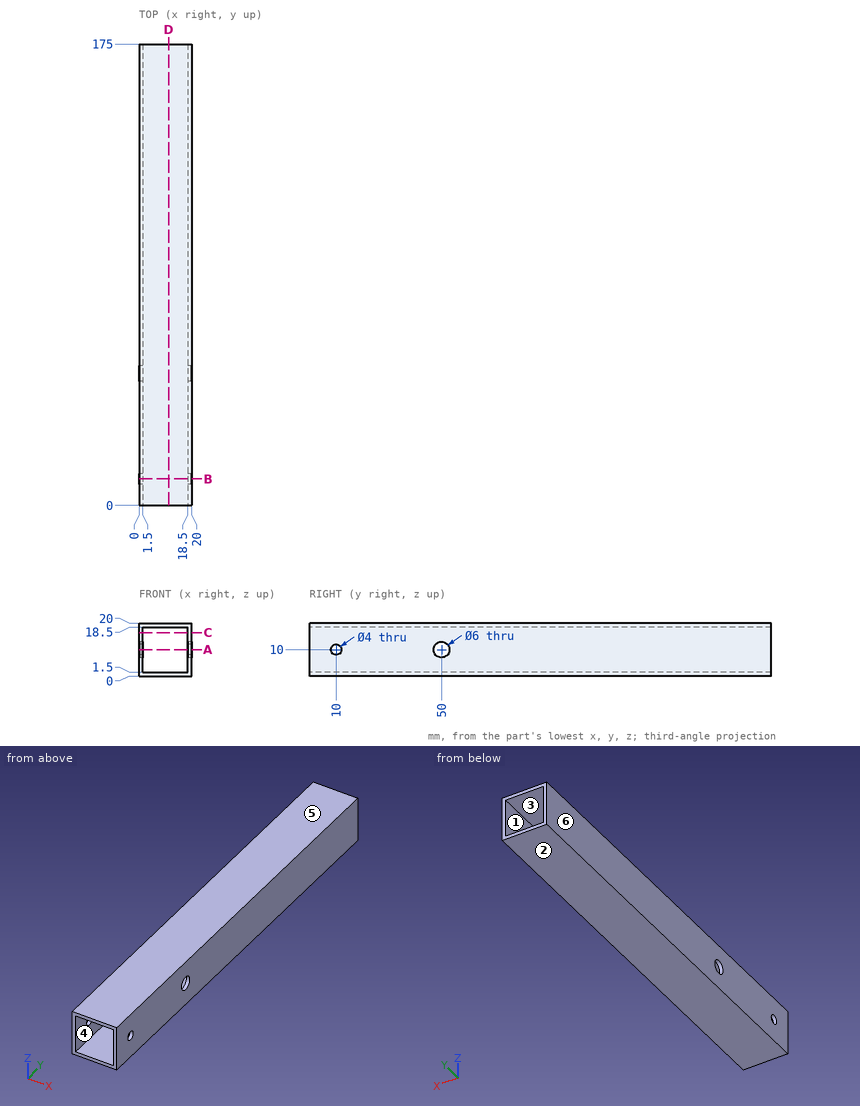
Can you work these out from the drawing? Everything is in mm from the part's minimum corner. A direction names the side the tool comes from. Coordinates: 2 decimals unless noted, no trailing zeros. Loops run counter-clockwise (first coordinate to the right, second up) from the corner with the lowest first, then second, coordinate; pieces in that order, holes last. Notation, with made-up numbers: M 2.25,-24 L 33.25,-24 A10 ccw 33.25,-19 Z; hole C 73.25,87 d10. An arc over 180 degrees is marked long. Put each result on its own line as item: value. Start each with the question number.
(1) Thinking about a two-plate mould opening in Z: for the marked faces 3, 4, 5 and 6, which applies, pulls with the +Z half, pulls with the -Z half, needs draft (parallel to the pull), parting line crosses it, or undercut?
(2) I need wall thicknesses on line 1 (Z direction, x = 0.3, y = 50); line 2 (Z direction, x = 1.75, y = 120). Which ranges of each line are inside material? Lowest first, please. Write a range as from..to.
(3) Suppose I cut it at A-A on z = 10. Please give me the cut outline in (x, y), then the cut area to 3 significant figures.
(4) Suppose I cut it at B-B on y = 10. Please give me the cut outline in (x, z), then the cut area to 3 significant figures.
(5) Suppose I cut it at C-C on z = 16.5. Please give me the cut outline in (x, y).
(6) Suppose I cut it at D-D on x = 11.25. Please give me the cut outline in (y, z), then the cut area to 3 significant figures.
(7) For the marked faces 1 and 2, which set-ups out of +Z, -Z, +X, -X, +Y, -Y let a thin tool reach every point of the face, with its end or its side?
(8) Will this pin go through, and if not, where does the flat tip stop? P1, Ø3.5, axis at y = 10, z = 10, coming from the +X side.
Solutions:
1. face 3: undercut
1. face 4: undercut
1. face 5: pulls with the +Z half
1. face 6: needs draft
2. line 1: z = 0..7, 13..20
2. line 2: z = 0..1.5, 18.5..20
3. outline: M 0,0 L 1.5,0 L 1.5,8 L 0,8 Z; M 0,12 L 1.5,12 L 1.5,47 L 0,47 Z; M 0,53 L 1.5,53 L 1.5,175 L 0,175 Z; M 18.5,0 L 20,0 L 20,8 L 18.5,8 Z; M 18.5,12 L 20,12 L 20,47 L 18.5,47 Z; M 18.5,53 L 20,53 L 20,175 L 18.5,175 Z
3. area: 495 mm2
4. outline: M 0,0 L 20,0 L 20,8 L 18.5,8 L 18.5,1.5 L 1.5,1.5 L 1.5,8 L 0,8 Z; M 0,12 L 1.5,12 L 1.5,18.5 L 18.5,18.5 L 18.5,12 L 20,12 L 20,20 L 0,20 Z
4. area: 99.0 mm2
5. outline: M 0,0 L 1.5,0 L 1.5,175 L 0,175 Z; M 18.5,0 L 20,0 L 20,175 L 18.5,175 Z
6. outline: M 0,0 L 175,0 L 175,1.5 L 0,1.5 Z; M 0,18.5 L 175,18.5 L 175,20 L 0,20 Z
6. area: 525 mm2
7. face 1: +Y, -Y
7. face 2: -Z, +X, -X, +Y, -Y
8. P1: passes through
